The model under review builds one solid part; all positions refer to its coordinate system, in mm. A direction names the side the tool comes from. Round coordinates to 2 decimals unless told otherwise and drop trailing zeros. Order: outer loops, then holes, each group sorted by start corner. A loop starts at its lowest first (then second) coordinate and runs counter-clockwise, first axis right, second up. Notation, with made-up numbers: M 65,-5 L 122,-5 A7 cw 122,7 Z; hole C 62,8.25 d3. An arc over 180 degrees is marked long. Use a Markdown table: item, result. Add a question column.
1. Consider section A-A on z = -5. State the section outline as (x, y) points (3 decimals), then the cut area to 3 significant figures.
2. To check wall thickness, follow probe 1 along X at (y, z) = (4.75, -5); probe 2 along X at (y, z) = (3.8, 5); probe 3 along Y at (x, z) = (-14, -3.5) (3 decimals). State the ranges of each line that lie inside material, in increasing order.
3. Consider section B-B on y = 3.75. State the section outline as (x, z) points.
4. Consider section D-D on z = 0. State the section outline as (x, y) points (3 decimals).
5. For faces 1 (the cylindrical face through (19.67, 4.64, -0.14)), 2 (the flat face through (25, 5.175, 0)), 3 (the flat face through (24, 3.175, 0)), list the 3-axis set-ups (+Z, -Z, +X, -X, +Y, -Y) from which the entire face can be reached by the end or side of a thin tool; tool diameter is ignored.
6. Consider section C-C on x = 9.95. State the section outline as (y, z) points (3 decimals).
7. Insertion check: P1, Ø2.5, axis at x = 22.5, z = 4, coming from the -Y side (3 decimals); P2, Ø1, axis at y = 6, z = -2, coming from the -X side; P3, Ø2, axis at x = 11, y = 5, coming from the +Z side; P4, Ø2.5, axis at y = 2, z = -2, coming from the -X side. Each pin has a flat end and moves straight along its axis. Give the tip position at first contact, or say it passes through.
8. The part is to be moulded in two halves that separate along X. For faces 4 (the flat face through (0, 0, 0)), 5 (the cylindrical face through (-19.625, 4.609, -0.141)), 6 (the flat face through (-20.05, 2, 0)), say which applies: +X half, -X half, draft (parallel to the pull), parting line (faces both ways), or undercut.
from build123d import *

# Parameters (mm, degrees)
SKETCH1_W            = 40.1
SKETCH1_H            = 20.1
BOSS_EXTRUDE1_DEPTH  = 3.175
SKETCH2_W            = 1.5
SKETCH2_H            = 20.1
BOSS_EXTRUDE2_DEPTH  = 2
SKETCH3_W            = 20.1
SKETCH3_H            = 2
BOSS_EXTRUDE3_DEPTH  = 8
SKETCH4_R            = 2
CUT_EXTRUDE1_DEPTH   = 30.964739695
FILLET1_R            = 3
FILLET2_R            = 3
FILLET1_OF_MIRROR2_R = 3
FILLET2_OF_MIRROR2_R = 3
SKETCH5_R            = 3
BOSS_EXTRUDE4_DEPTH  = 5


with BuildPart() as part:
    # Sketch1 → Boss-Extrude1 (new body)
    with BuildSketch(Plane(origin=(0, 0, 0), x_dir=(1, 0, 0), z_dir=(0, 1, 0))):
        Rectangle(SKETCH1_W, SKETCH1_H)
    extrude(amount=BOSS_EXTRUDE1_DEPTH)

    # Sketch2 → Boss-Extrude2 (add)
    with BuildSketch(Plane(origin=(0, 3.175, 0), x_dir=(1, 0, 0), z_dir=(0, 1, 0))):
        with Locations((19.3, 0)):
            Rectangle(SKETCH2_W, SKETCH2_H)
    boss_extrude2 = extrude(amount=BOSS_EXTRUDE2_DEPTH)

    # Sketch3 → Boss-Extrude3 (add)
    with BuildSketch(Plane(origin=(20.05, 0, 0), x_dir=(0, 0, -1), z_dir=(1, 0, 0))):
        with Locations((0, 4.175)):
            Rectangle(SKETCH3_W, SKETCH3_H)
    boss_extrude3 = extrude(amount=BOSS_EXTRUDE3_DEPTH)

    # Sketch4 → Cut-Extrude1 (cut, symmetric)
    with BuildSketch(Plane.XZ.offset(-3.175)):
        with Locations(Location((25.05, 5, 0), (0, 0, 270))):
            Circle(SKETCH4_R)
        with Locations(Location((25.05, -5, 0), (0, 0, 270))):
            Circle(SKETCH4_R)
    cut_extrude1 = extrude(amount=CUT_EXTRUDE1_DEPTH, both=True, mode=Mode.SUBTRACT)

    # Fillet1
    # the kernel refuses this fillet: 3 mm, written as the material it takes off along each edge
    with BuildSketch(Plane(origin=(18.55, 5.175, -17.121067812), x_dir=(0, -1, 0), z_dir=(0, 0, 1))) as fillet1_piece_1:
        with BuildLine():
            CenterArc((3, 2.828427125), FILLET1_R, 180, 70.528779366)
            Line((0, 2.828427125), (-0.06, 2.828427125))
            Line((-0.06, 2.828427125), (-0.06, 0))
            Line((-0.06, 0), (0, -0.06))
            ThreePointArc((0, -0.06), (1, -0.06), (1.98, -0.056568542))
            Line((1.98, -0.056568542), (2, 0))
        make_face()
    extrude(amount=34.242135624, mode=Mode.SUBTRACT)

    # Fillet2
    fillet2_edges = [part.edges().sort_by_distance(p)[0] for p in [
        (28.05, 4.175, 10.05),
        (28.05, 4.175, -10.05),
    ]]
    fillet(fillet2_edges, radius=FILLET2_R)

    # Mirror2: Boss-Extrude2, Boss-Extrude3, Cut-Extrude1 across plane
    add(boss_extrude2.mirror(Plane(origin=(0, 0, 0), x_dir=(0, 0, 1), z_dir=(1, 0, 0))))
    add(boss_extrude3.mirror(Plane(origin=(0, 0, 0), x_dir=(0, 0, 1), z_dir=(1, 0, 0))))
    add(cut_extrude1.mirror(Plane(origin=(0, 0, 0), x_dir=(0, 0, 1), z_dir=(1, 0, 0))), mode=Mode.SUBTRACT)

    # Fillet1 of Mirror2
    # the kernel refuses this fillet: 3 mm, written as the material it takes off along each edge
    with BuildSketch(Plane(origin=(-18.55, 5.175, -17.121067812), x_dir=(-1, 0, 0), z_dir=(0, 0, 1))) as fillet1_of_mirror2_piece_1:
        with BuildLine():
            CenterArc((2.828427125, 3), FILLET1_OF_MIRROR2_R, 199.471220634, 70.528779366)
            Line((0, 2), (-0.056568542, 1.98))
            ThreePointArc((-0.056568542, 1.98), (-0.06, 1), (-0.06, 0))
            Line((-0.06, 0), (0, -0.06))
            Line((0, -0.06), (2.828427125, -0.06))
            Line((2.828427125, -0.06), (2.828427125, 0))
        make_face()
    extrude(amount=34.242135624, mode=Mode.SUBTRACT)

    # Fillet2 of Mirror2
    fillet2_of_mirror2_edges = [part.edges().sort_by_distance(p)[0] for p in [
        (-28.05, 4.175, 10.05),
        (-28.05, 4.175, -10.05),
    ]]
    fillet(fillet2_of_mirror2_edges, radius=FILLET2_OF_MIRROR2_R)

    # Sketch5 → Boss-Extrude4 (add)
    with BuildSketch(Plane(origin=(0, 3.175, 0), x_dir=(1, 0, 0), z_dir=(0, 1, 0))):
        with Locations(Location((9.95, 0, 0), (0, 0, 90))):
            Circle(SKETCH5_R)
    extrude(amount=BOSS_EXTRUDE4_DEPTH)


solid = part.part
Answer block:
| question | item | result |
|---|---|---|
| 1 | outline | M -28.05,3.175 L -27.05,3.175 L -27.05,5.175 L -28.05,5.175 Z; M -23.05,3.175 L -20.05,3.175 L -20.05,0 L 20.05,0 L 20.05,3.175 L 23.05,3.175 L 23.05,5.175 L 21.378,5.175 A3 ccw 18.55,3.175 L -18.55,3.175 A3 ccw -21.378,5.175 L -23.05,5.175 Z; M 27.05,3.175 L 28.05,3.175 L 28.05,5.175 L 27.05,5.175 Z |
| 1 | area | 146 mm^2 |
| 2 | probe 1 | -28.05 to -27.05, -23.05 to -19.84, 19.84 to 23.05, 27.05 to 28.05 |
| 2 | probe 2 | -28.05 to -27.05, -23.05 to -18.86, 18.86 to 23.05, 27.05 to 28.05 |
| 2 | probe 3 | 0 to 3.175 |
| 3 | outline | M -28.05,-7.05 A3 ccw -25.05,-10.05 L -18.83,-10.05 L -18.83,10.05 L -25.05,10.05 A3 ccw -28.05,7.05 Z; C 9.95,0 d6; M 18.83,-10.05 L 25.05,-10.05 A3 ccw 28.05,-7.05 L 28.05,7.05 A3 ccw 25.05,10.05 L 18.83,10.05 Z; hole C -25.05,-5 d4; hole C -25.05,5 d4; hole C 25.05,-5 d4; hole C 25.05,5 d4 |
| 4 | outline | M -28.05,3.175 L -20.05,3.175 L -20.05,0 L 20.05,0 L 20.05,3.175 L 28.05,3.175 L 28.05,5.175 L 21.378,5.175 A3 ccw 18.55,3.175 L 12.95,3.175 L 12.95,8.175 L 6.95,8.175 L 6.95,3.175 L -18.55,3.175 A3 ccw -21.378,5.175 L -28.05,5.175 Z |
| 5 | face 1 | +Z, -Z, +Y |
| 5 | face 2 | +Z, -Z, +X, +Y |
| 5 | face 3 | +Z, -Z, +X, -Y |
| 6 | outline | M 0,-10.05 L 3.175,-10.05 L 3.175,-3 L 8.175,-3 L 8.175,3 L 3.175,3 L 3.175,10.05 L 0,10.05 Z |
| 7 | P1 | y = 3.175 |
| 7 | P2 | x = 7.35 |
| 7 | P3 | z = 3 |
| 7 | P4 | x = -28.05 |
| 8 | face 4 | draft |
| 8 | face 5 | undercut |
| 8 | face 6 | -X half |
